Work out the finished part from the listing and answer in its coordinate system (mm). A direction names the side the tool comes from. Give positions to 0.01 mm unless a question says otherwise; leave off trailing zeros. Write each loop counter-clockwise with the first axis right and the second up, starting at its lowest first coordinate (ties: lowest second). Pieces come first, ordered by that corner, then holes. Notation, with made-up numbers: (86.5, 40) -> (118.5, 40) arc R36 ccw to (118.5, 75) -> close; hole circle Ø9 at (18.5, -26.5). An arc over 180 degrees is marked (long way). Use a Markdown table: item, result. Add a question column.
Q1. Section C-C, the plane x = 86.5 is taken. Give the vertices of the cut face in (y, z), plus the area to 3 significant figures.
Q2. Section D-D, the plane z = 18.5 is taken. Give the vertices of the cut face in (x, y).
Q3. Section B-B, the plane z = -6 is taken. Give the vertices of the cut face in (x, y), plus the area to 3 significant figures.
Q4. Section A-A, the plane x = 0 is taken. Give the vertices of the cut face in (y, z), plus the area to 3 significant figures.
Q5. Each of these flat-tipped pins is pushed along its axis until it touches: pin 1 Ø2 at (y, z) = (6, 2.5) entering from +X; pin 2 Ø1 at (y, z) = (7.5, 19.5) entering from -X; pin 3 Ø3 at (x, y) = (57.5, 4) entering from +Z. Where does it stop, or does it pass through?
Q6. For a pull along X with two mould halves and no side action, classify faces 1 (the face through (17.24, 4.93, 17.64)), 2 (the face through (20, 10, 0)), 3 (the face through (143.22, 4.93, 12.28)) as pulls with the +X half, pulls with the -X half, needs draft (parallel to the pull), parting line crosses it, or undercut.
Q7. Consider line 1 (X direction, y = 3, z = 20); line 2 (Z direction, x = 53.5, y = 4.5); line 3 (X direction, y = 2.5, z = 13). Determine where each line is inside the solid, lowest interval first.
Q8. For faces 4 (the face through (68, 2, 15)), 5 (the face through (114.687, 4.93, 11.99)), 6 (the face through (68, 2.5, 7)), 7 (the face through (39, 0, 7)), determine the directions among +Z, -Z, +X, -X, +Y, -Y from which every point of the face is accessible in a straight line to the end or side of a thin tool.
Autodesk Fusion 360 part; units mm, degrees
sketch "Sketch1" plane through (0, 0, 0) normal (0, 1, 0) x (1, 0, 0)
  line L0 (139.8981, -22.5) -> (146.6336, -1.7705)
  line L1 (146.6336, -1.7705) -> (129, 11.041)
  line L2 (129, 11.041) -> (111.3664, -1.7705)
  line L3 (111.3664, -1.7705) -> (118.1019, -22.5)
  line L4 (118.1019, -22.5) -> (139.8981, -22.5)
  line L5 (11.547, -27.5) -> (23.094, -7.5)
  line L6 (23.094, -7.5) -> (11.547, 12.5)
  line L7 (11.547, 12.5) -> (-11.547, 12.5)
  line L8 (-11.547, 12.5) -> (-23.094, -7.5)
  line L9 (-23.094, -7.5) -> (-11.547, -27.5)
  line L10 (-11.547, -27.5) -> (11.547, -27.5)
  circle A0 centre (0, -7.5) radius 30
  circle A1 centre (129, -7.5) radius 22.5
  line L11 (38.4299, -12.3139) -> (98.4299, -12.3139)
  line L12 (103.4299, -7.3139) -> (103.4299, -7.3123)
  line L13 (98.4299, -2.3142) -> (38.479, -2.3142)
  line L14 (38.7, -2.3142) -> (38.479, -2.3142)
  arc A2 (38.479, -2.3142) -> (38.4299, -12.3139) centre (38.4299, -7.3139) ccw
  arc A3 (103.4299, -7.3123) -> (98.4299, -2.3142) centre (98.4299, -7.3142) ccw
  arc A4 (98.4299, -12.3139) -> (103.4299, -7.3139) centre (98.4299, -7.3139) ccw
  line L15 (28.6408, -15) -> (109.0777, -15)
  line L16 (109.0777, 0) -> (28.6408, 0)
  point P0 (0, -7.5)
  point P1 (129, -7.5)
  point P2 (103.4299, -12.3139)
  dimension "d2" = 20
  dimension "d3" = 60
  dimension "d4" = 45
  dimension "d7" = 5
extrude "Extrude1" add sketch "Sketch1" along normal blind 10 contours A0 | A1 makes body 1 at (-13.6863, 6.6667, 34.1962) makes body 2 at (151.3882, 3.3333, 9.7403)
extrude "Extrude2" add sketch "Sketch1" along normal blind 5 contours A0 A1 L15 L16 bodies 1 2
extrude "Extrude3" add sketch "Sketch1" along normal blind 2.5 contours L11 L13 L14 A2 A3 A4 bodies 1
Result set:
| question | item | result |
|---|---|---|
| 1 | outline | (0, 0) -> (5, 0) -> (5, 2.31) -> (2.5, 2.31) -> (2.5, 12.31) -> (5, 12.31) -> (5, 15) -> (0, 15) -> close |
| 1 | area | 50.0 mm2 |
| 2 | outline | (-27.91, 0) -> (-16.74, 0) -> (-16.74, 10) -> (-27.91, 10) -> close; (16.74, 0) -> (27.91, 0) -> (27.91, 10) -> (16.74, 10) -> close; (109.37, 0) -> (116.8, 0) -> (116.8, 10) -> (109.37, 10) -> close; (141.2, 0) -> (148.63, 0) -> (148.63, 10) -> (141.2, 10) -> close |
| 3 | outline | (-26.79, 0) -> (-15.3, 0) -> (-15.3, 10) -> (-26.79, 10) -> close; (15.3, 0) -> (26.79, 0) -> (26.79, 10) -> (15.3, 10) -> close; (111, 0) -> (122.06, 0) -> (122.06, 10) -> (111, 10) -> close; (135.94, 0) -> (147, 0) -> (147, 10) -> (135.94, 10) -> close |
| 3 | area | 451 mm2 |
| 4 | outline | (0, -22.5) -> (10, -22.5) -> (10, -12.5) -> (0, -12.5) -> close; (0, 27.5) -> (10, 27.5) -> (10, 37.5) -> (0, 37.5) -> close |
| 4 | area | 200 mm2 |
| 5 | pin 1 | stops at x = 151.14 |
| 5 | pin 2 | stops at x = -27.71 |
| 5 | pin 3 | stops at z = 15 |
| 6 | face 1 | undercut |
| 6 | face 2 | needs draft |
| 6 | face 3 | undercut |
| 7 | line 1 | x = -27.27 to -15.88, 15.88 to 27.27, 110.29 to 117.29, 140.71 to 147.71 |
| 7 | line 2 | z = 0 to 2.31, 12.31 to 15 |
| 7 | line 3 | x = -29.49 to -19.92, 19.92 to 115.02, 142.98 to 150.82 |
| 8 | face 4 | +Z, +Y, -Y |
| 8 | face 5 | +Y, -Y |
| 8 | face 6 | +Y |
| 8 | face 7 | +Z, -Z, +X, -X, -Y |
